Design review of the part built by this model. Coordinates are the model's own, in mm. A direction names the side the tool comes from. Coordinates: 2 decimals unless noted, no trailing zeros. Write each loop counter-clockwise with the first axis right and the second up, starting at its lowest first coordinate (ties: lowest second). Pieces come first, ordered by that corner, then holes. Notation, with made-up numbers: (-39.5, 5.5) - (-8.5, 5.5) arc R5 cw to (-8.5, 11.5) - close; hole circle Ø7 at (49.25, -12). An arc over 180 degrees is marked (long way). Answer as a JSON object with one key per item and string values.
```python
from build123d import *

# Parameters (mm, degrees)
SKETCH1_W           = 300
SKETCH1_H           = 300
BOSS_EXTRUDE1_DEPTH = 40
FILLET1_R           = 20
SKETCH2_W           = 249
SKETCH2_H           = 249
BOSS_EXTRUDE2_DEPTH = 15
SKETCH3_W           = 140
SKETCH3_H           = 60
CUT_EXTRUDE1_DEPTH  = 25
SKETCH4_R           = 10
CUT_EXTRUDE2_DEPTH  = 428.814212013


with BuildPart() as part:
    # Sketch1 → Boss-Extrude1 (new body)
    with BuildSketch(Plane(origin=(0, 0, 0), x_dir=(1, 0, 0), z_dir=(0, 1, 0))):
        with Locations((150, 150)):
            Rectangle(SKETCH1_W, SKETCH1_H)
    extrude(amount=BOSS_EXTRUDE1_DEPTH)

    # Fillet1
    fillet1_edges = [part.edges().sort_by_distance(p)[0] for p in [
        (300, 40, -150),
        (150, 40, -300),
        (0, 40, -150),
        (150, 40, 0),
        (0, 20, -300),
        (300, 20, -300),
        (300, 20, 0),
        (0, 20, 0),
    ]]
    fillet(fillet1_edges, radius=FILLET1_R)

    # Sketch2 → Boss-Extrude2 (add)
    with BuildSketch(Plane.XZ):
        with Locations((150, -150)):
            Rectangle(SKETCH2_W, SKETCH2_H)
    extrude(amount=BOSS_EXTRUDE2_DEPTH)

    # Sketch3 → Cut-Extrude1 (cut)
    with BuildSketch(Plane.XZ.offset(15)):
        with Locations((150, -90)):
            Rectangle(SKETCH3_W, SKETCH3_H)
        with Locations((150, -210)):
            Rectangle(SKETCH3_W, SKETCH3_H)
    extrude(amount=-CUT_EXTRUDE1_DEPTH, mode=Mode.SUBTRACT)

    # Sketch4 → Cut-Extrude2 (cut, through all)
    with BuildSketch(Plane(origin=(0, -15, 0), x_dir=(-1, 0, 0), z_dir=(0, -1, 0))):
        with Locations(Location((-150, 150, 0), (0, 0, 90))):
            Circle(SKETCH4_R)
    extrude(amount=-CUT_EXTRUDE2_DEPTH, mode=Mode.SUBTRACT)


solid = part.part
```
(1) For pin 1 (7.5 mm diameter, centred on y = -6.5, z = -141, fed in from +X); pin 2 (12.5 mm diameter, centred on y = -7, z = -83, fed in from -X); pin 3 (3 mm diameter, centred on x = 138.5, y = 23.5, fed in from -Z), all flat-tipped, find the tip position at first contact; note any pin that passes through.
Solved:
{"pin 1": "stops at x = 274.5", "pin 2": "stops at x = 25.5", "pin 3": "stops at z = -299.9"}
(2) To check wall thickness, follow line 1 (Z direction, x = 88, y = 8); line 2 (X direction, y = 6, z = -150); line 3 (X direction, y = 21.5, z = -45). State the ranges of each line that lie inside material, in increasing order. Write a range as from..to.
Solved:
{"line 1": "z = -300..-240, -180..-120, -60..0", "line 2": "x = 0..140, 160..300", "line 3": "x = 0.06..299.94"}
(3) Take a section at B-B, the plane z = -150. Write out the cut boundary in (x, y).
Solved:
{"outline": "(0, 0) - (25.5, 0) - (25.5, -15) - (140, -15) - (140, 40) - (20, 40) arc R20 ccw to (0, 20) - close; (160, -15) - (274.5, -15) - (274.5, 0) - (300, 0) - (300, 20) arc R20 ccw to (280, 40) - (160, 40) - close"}
(4) Take a section at D-D, the plane y = 35. Write out the cut boundary in (x, z), and give its area (3 significant figures).
Solved:
{"outline": "(6.77, -280) arc R13.23 ccw to (20, -293.23) - (280, -293.23) arc R13.23 ccw to (293.23, -280) - (293.23, -20) arc R13.23 ccw to (280, -6.77) - (20, -6.77) arc R13.23 ccw to (6.77, -20) - close; hole circle Ø20 at (150, -150)", "area": "81,600 mm^2"}
(5) Take a section at C-C, the plane x = 150. Write out the cut boundary in (y, z), and give its area (3 significant figures).
Solved:
{"outline": "(-15, -274.5) - (0, -274.5) - (0, -300) - (20, -300) arc R20 ccw to (40, -280) - (40, -160) - (-15, -160) - (-15, -180) - (10, -180) - (10, -240) - (-15, -240) - close; (-15, -140) - (40, -140) - (40, -20) arc R20 ccw to (20, 0) - (0, 0) - (0, -25.5) - (-15, -25.5) - (-15, -60) - (10, -60) - (10, -120) - (-15, -120) - close", "area": "11,500 mm^2"}
(6) The part is to be moulded in two halves that separate along Z. For faces 4 (the face through (148, 10, 0)), 5 (the face through (149, 10, -90)), 6 (the face through (294.297, 10.14, -293.986)), say which applies: pulls with the +Z half, pulls with the -Z half, needs draft (parallel to the pull), parting line crosses it, or undercut.
Solved:
{"face 4": "pulls with the +Z half", "face 5": "undercut", "face 6": "pulls with the -Z half"}
(7) Tool access review of faces 1 (the face through (148, -7, -25.5)), 2 (the face through (149, -3, -120)), 3 (the face through (274.5, -7, -152)): name each direction out of +Z, -Z, +X, -X, +Y, -Y from which nothing blocks a thin tool from reaching the whole face with its end or side.
Solved:
{"face 1": "+Z, +X, -X, -Y", "face 2": "-Y", "face 3": "+Z, -Z, +X, -Y"}
(8) Take a section at A-A, the plane x = 207.5. Write out the cut boundary in (y, z), and give its area (3 significant figures).
Solved:
{"outline": "(-15, -274.5) - (0, -274.5) - (0, -300) - (20, -300) arc R20 ccw to (40, -280) - (40, -20) arc R20 ccw to (20, 0) - (0, 0) - (0, -25.5) - (-15, -25.5) - (-15, -60) - (10, -60) - (10, -120) - (-15, -120) - (-15, -180) - (10, -180) - (10, -240) - (-15, -240) - close", "area": "12,600 mm^2"}
